from build123d import *

# Parameters (mm, degrees)
F1_DEPTH  = 38.1
F2_W      = 25.4
F2_H      = 25.4
F3_DEPTH  = 31.75
F4_W      = 12.7
F4_H      = 12.7
F5_DEPTH  = 12.7
F7_DEPTH  = 25.4
F9_DEPTH  = 25.4
F10_R     = 6.35
F11_DEPTH = 25.4
F12_R     = 3.175
F13_DEPTH = 25.4
F15_DEPTH = 25.4


with BuildPart() as f1:
    # F0 (on Front) → F1 (new body)
    with BuildSketch(Plane.XZ):
        Polygon((-80.9037027093, 0), (0, 0), (0, 6.35), (-55.5037027093, 6.35), (-55.5037027093, 38.1), (-80.9037027093, 38.1), align=None)
    extrude(amount=F1_DEPTH)

    # F2 (on face) → F3 (cut)
    with BuildSketch(Plane.XY.offset(38.1)):
        with Locations((-68.2037027093, -25.4)):
            Rectangle(F2_W, F2_H)
    extrude(amount=-F3_DEPTH, mode=Mode.SUBTRACT)

    # F4 (on face) → F5 (join)
    with BuildSketch(Plane.XY.offset(6.35)):
        with Locations((-49.1537027093, -6.35)):
            Rectangle(F4_W, F4_H)
    extrude(amount=F5_DEPTH)

    # F6 (on face) → F7 (cut)
    with BuildSketch(Plane(origin=(0, 0, 0), x_dir=(-1, 0, 0), z_dir=(0, 1, 0))):
        with BuildLine():
            ThreePointArc((42.8037027093, 6.35), (51.7839588303, 10.0697438789), (55.5037027093, 19.05))
            Line((55.5037027093, 19.05), (42.8037027093, 19.05))
            Line((42.8037027093, 19.05), (42.8037027093, 6.35))
        make_face()
    extrude(amount=-F7_DEPTH, mode=Mode.SUBTRACT)

    # F8 (on face) → F9 (cut)
    with BuildSketch(Plane.XZ.offset(12.7)):
        with BuildLine():
            ThreePointArc((-80.9037027093, 25.4), (-77.1839588303, 34.3802561211), (-68.2037027093, 38.1))
            Line((-68.2037027093, 38.1), (-80.9037027093, 38.1))
            Line((-80.9037027093, 38.1), (-80.9037027093, 25.4))
        make_face()
        with BuildLine():
            ThreePointArc((-68.2037027093, 38.1), (-59.2234465882, 34.3802561211), (-55.5037027093, 25.4))
            Line((-55.5037027093, 25.4), (-55.5037027093, 38.1))
            Line((-55.5037027093, 38.1), (-68.2037027093, 38.1))
        make_face()
    extrude(amount=-F9_DEPTH, mode=Mode.SUBTRACT)

    # F10 (on face) → F11 (cut)
    with BuildSketch(Plane.XZ.offset(12.7)):
        with Locations((-68.2037027093, 25.4)):
            Circle(F10_R)
    extrude(amount=-F11_DEPTH, mode=Mode.SUBTRACT)

    # F12 (on face) → F13 (cut)
    with BuildSketch(Plane.XY.offset(6.35)):
        with Locations((-9.525, -9.525)):
            Circle(F12_R)
        with Locations((-9.525, -28.575)):
            Circle(F12_R)
        with Locations((-71.3787027093, -28.575)):
            Circle(F12_R)
    extrude(amount=-F13_DEPTH, mode=Mode.SUBTRACT)

    # F14 (on face) → F15 (cut)
    with BuildSketch(Plane.XY.offset(6.35)):
        with BuildLine():
            Line((-80.9037027093, -38.1), (-74.5537027093, -38.1))
            ThreePointArc((-74.5537027093, -38.1), (-79.0438307698, -36.2401280605), (-80.9037027093, -31.75))
            Line((-80.9037027093, -31.75), (-80.9037027093, -38.1))
        make_face()
        with BuildLine():
            ThreePointArc((0, -31.75), (-1.8598719244, -36.2401280455), (-6.3499999575, -38.1))
            Line((-6.3499999575, -38.1), (0, -38.1))
            Line((0, -38.1), (0, -31.75))
        make_face()
    extrude(amount=-F15_DEPTH, mode=Mode.SUBTRACT)


solid = f1.part
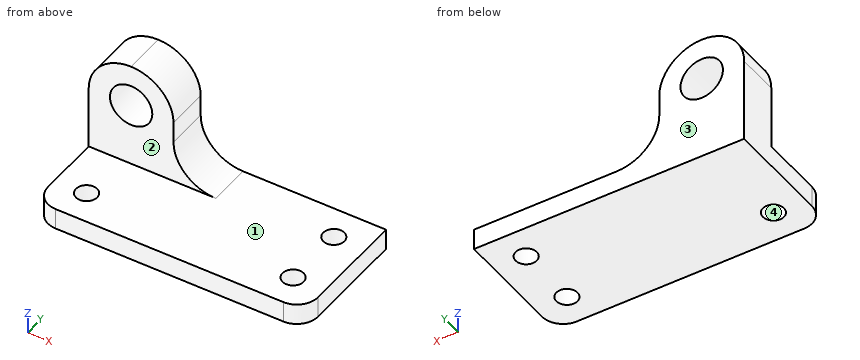
For this review, take the finished solid that the model builds, in its own axes (mm). Face numbers are marked on the shaded views. Give positions to 0.01 mm unless a question says otherwise; leave off trailing zeros. Loops run counter-clockwise (first coordinate to the right, second up) from the corner with the lowest first, then second, coordinate; pieces in that order, holes last. Notation, with made-up numbers: M 13.25,72.25 L 57.25,72.25 A20 ccw 57.25,108.25 Z; hole C 21.25,78 d8. An arc over 180 degrees is marked long. Put each result on its own line as item: value. Start each with the question number.
(1) Add section B-B, the plane x = -67. Write out the cut boundary in (y, z), then the cut area to 3 significant figures.
(2) For pin 1 (5 mm diameter, centred on x = -46.5, y = -8.5, fed in from +Z); pin 2 (10 mm diameter, centred on x = -9.525, y = -9.525, fed in from +Z); pin 3 (20.5 mm diameter, centred on x = -68.2, z = 25.4, fed in from -Y), all flat-tipped, find the tip position at first contact; note any pin that passes through.
(3) Add section C-C, the plane z = 5. Write out the cut boundary in (x, y) (3 decimals), then the cut area to 3 significant figures.
(4) Add section A-A, the plane y = -8. Write out the cut boundary in (x, z), then the cut area to 3 significant figures.
(5) Wall thickness on L1, parallel to Y at x = -64.5, z = 33.5; L2, parallel to Z at x = -34.5, y = -23; L3, parallel to X at y = -26.5, z = 5: over which ranges is each line inside the solid? List them lowest first.
(6) The part is to be moulded in two halves that separate along Y. For the marked faces 1, 2, 3 and 4, say which applies: +Y half, -Y half, draft (parallel to the pull), parting line (faces both ways), or undercut.
(7) Add section D-D, the plane x = -26. Write out the cut boundary in (y, z).
Result:
1. outline: M -38.1,0 L 0,0 L 0,19.17 L -12.7,19.17 L -12.7,6.35 L -38.1,6.35 Z; M -12.7,31.63 L 0,31.63 L 0,38.04 L -12.7,38.04 Z
1. area: 486 mm^2
2. pin 1: stops at z = 7.96
2. pin 2: stops at z = 6.35
2. pin 3: stops at y = -12.7
3. outline: M -80.904,-31.75 A6.35 ccw -74.554,-38.1 L -6.35,-38.1 A6.35 ccw 0,-31.75 L 0,0 L -80.904,0 Z; hole C -71.379,-28.575 d6.35; hole C -9.525,-28.575 d6.35; hole C -9.525,-9.525 d6.35
3. area: 2,970 mm^2
4. outline: M -80.9,0 L -12.31,0 L -12.31,6.35 L -42.8,6.35 A12.7 cw -55.5,19.05 L -55.5,25.4 A12.7 ccw -80.9,25.4 Z; M -6.74,0 L 0,0 L 0,6.35 L -6.74,6.35 Z; hole C -68.2,25.4 d12.7
4. area: 1,120 mm^2
5. L1: y = -12.7 to 0
5. L2: z = 0 to 6.35
5. L3: x = -80.9 to -73.78, -68.98 to -11.93, -7.12 to 0
6. face 1: draft
6. face 2: -Y half
6. face 3: +Y half
6. face 4: undercut
7. outline: M -38.1,0 L 0,0 L 0,6.35 L -38.1,6.35 Z
